from build123d import *

# Parameters (mm, degrees)
F1_DEPTH = 65
F3_SIZE  = 2
F2_R     = 3
F4_DEPTH = 12


with BuildPart() as f1:
    # F0 (on Front) → F1 (new body)
    with BuildSketch(Plane.XZ):
        with BuildLine():
            ThreePointArc((-5.75, -11.098986), (0, 12.5), (5.75, -11.098986))
            Line((5.75, -11.098986), (9.900611, -20))
            Line((9.900611, -20), (30, -20))
            Line((30, -20), (30, -11.098986))
            Line((30, -11.098986), (30, 27))
            Line((30, 27), (15, 27))
            Line((15, 27), (13, 25))
            Line((13, 25), (7, 25))
            Line((7, 25), (5, 27))
            Line((5, 27), (0, 27))
            Line((0, 27), (-5, 27))
            Line((-5, 27), (-7, 25))
            Line((-7, 25), (-13, 25))
            Line((-13, 25), (-15, 27))
            Line((-15, 27), (-30, 27))
            Line((-30, 27), (-30, -11.098986))
            Line((-30, -11.098986), (-30, -20))
            Line((-30, -20), (-9.900611, -20))
            Line((-9.900611, -20), (-5.75, -11.098986))
        make_face()
    extrude(amount=-F1_DEPTH)

    # F3
    f3_edges = [f1.edges().sort_by_distance(p)[0] for p in [
        (30, 32.5, 27),
        (-30, 32.5, 27),
    ]]
    chamfer(f3_edges, length=F3_SIZE)

    # F2 (on face) → F4 (cut)
    with BuildSketch(Plane.XY.offset(27)):
        with Locations((-20, 52.5)):
            Circle(F2_R)
        with Locations((-20, 12.5)):
            Circle(F2_R)
        with Locations((20, 52.5)):
            Circle(F2_R)
        with Locations((20, 12.5)):
            Circle(F2_R)
    extrude(amount=-F4_DEPTH, mode=Mode.SUBTRACT)


solid = f1.part
Read the model definition and answer for the solid it produces. Units are mm, in the model's axes. A direction names the side the tool comes from. Give positions to 0.01 mm unless a question says otherwise; leave off trailing zeros. Loops run counter-clockwise (first coordinate to the right, second up) from the corner with the lowest first, then second, coordinate; pieces in that order, holes last. Notation, with made-up numbers: (51.25, 14) - (96.25, 14) arc R11 cw to (96.25, 19) - close; hole circle Ø1 at (2.5, 83). An arc over 180 degrees is marked (long way). Answer as CSV lines item,"result". Start each with the question number.
1) Straight lines are drawn through the part: L1, parallel to Y at x = 20, z = 23; L2, parallel to X at y = 5.5, z = -0.5; L3, parallel to X at y = 62, z = 5. For each, find the intervals that lie inside material, in ascending order. Write a range as from..to.
2) Find section C-C (z = 17.5). Write down the section's boundary in (x, y).
3) Each of these flat-tipped pins is pushed along its axis until it touches: pin 1 Ø9.5 at (x, y) = (-20, 12.5) entering from +Z; pin 2 Ø3 at (x, y) = (11, 33) entering from +Z; pin 3 Ø3 at (x, y) = (20.5, 13.5) entering from +Z. Where does it stop, or does it pass through?
4) Which of the six approach directions +Z, -Z, +X, -X, +Y, -Y give full straight-line access (tool end or side, diameter ignored) to faces 1 (the face through (20, 13, 15)), 2 (the face through (-7.854, 32.045, -15.612)), 3 (the face through (-10, 32, 25))?
5) Find section D-D (x = 11.5). Write down the section's boundary in (y, z).
6) Determine the mould class of faces 4 (the face through (22, 32, 27)), 5 (the face through (30, 32, 2)), 6 (the face through (-0.47, 32.04, 12.49)) for opening direction X: released by +X, released by -X, zero draft, split by the parting line, or undercut.
7) Find section A-A (z = 0). Write down the section's boundary in (x, y).
8) Find section B-B (y = 52.5). Write down the section's boundary in (x, z), then the cut area to 3 significant figures.
Findings below:
1,L1,"0..9.5, 15.5..49.5, 55.5..65"
1,L2,"-30..-12.49, 12.49..30"
1,L3,"-30..-11.46, 11.46..30"
2,outline,"(-30, 0) - (30, 0) - (30, 65) - (-30, 65) - close; hole circle Ø6 at (-20, 12.5); hole circle Ø6 at (-20, 52.5); hole circle Ø6 at (20, 12.5); hole circle Ø6 at (20, 52.5)"
3,pin 1,"z = 27"
3,pin 2,"z = 25"
3,pin 3,"z = 15"
4,face 1,"+Z"
4,face 2,"-Z, +Y, -Y"
4,face 3,"+Z, +Y, -Y"
5,outline,"(0, -20) - (65, -20) - (65, -4.9) - (0, -4.9) - close; (0, 4.9) - (65, 4.9) - (65, 25) - (0, 25) - close"
6,face 4,"zero draft"
6,face 5,"released by +X"
6,face 6,"undercut"
7,outline,"(-30, 0) - (-12.5, 0) - (-12.5, 65) - (-30, 65) - close; (12.5, 0) - (30, 0) - (30, 65) - (12.5, 65) - close"
8,outline,"(-30, -20) - (-9.9, -20) - (-5.75, -11.1) arc R12.5 cw (long way) to (5.75, -11.1) - (9.9, -20) - (30, -20) - (30, 25) - (28, 27) - (23, 27) - (23, 15) - (17, 15) - (17, 27) - (15, 27) - (13, 25) - (7, 25) - (5, 27) - (-5, 27) - (-7, 25) - (-13, 25) - (-15, 27) - (-17, 27) - (-17, 15) - (-23, 15) - (-23, 27) - (-28, 27) - (-30, 25) - close"
8,area,"2,020 mm^2"
